For this review, take the finished solid that the model builds, in its own axes (mm). A direction names the side the tool comes from. Give positions to 0.01 mm unless a question says otherwise; leave off trailing zeros. Order: outer loops, then holes, each group sorted by start corner. A loop starts at its lowest first (then second) coordinate and runs counter-clockwise, first axis right, second up. Notation, with made-up numbers: (5, 30) - (35, 30) arc R14 ccw to (35, 35) - close; hole circle Ø6 at (54.5, -10.75). An arc over 180 degrees is marked (long way). Use a Markdown table: item, result. Add a question column.
1) We need section A-A on y = 1.55. Write out the cut boundary in (x, z).
2) Machinability: for faces 1 (the face through (8, 2, -7)), 2 (the face through (17, 2, -4)), 3 (the face through (18.5, -1, -5)), which of the approach directions +Z, -Z, +X, -X, +Y, -Y give a long, thin tool a straight path to every point of the face, cutting with its end or side? Answer none if there is none.
3) Clearance check with flat-ended pins moving along their axes: P1, Ø3, axis at x = 9, z = -13.5, coming from the -Y side; P2, Ø1, axis at y = 2, z = -6, coming from the -X side; P3, Ø5, axis at x = 13, z = -10.5, coming from the +Y side; P4, Ø0.8, axis at y = -1, z = -8, coming from the +X side. State where each tip first meets the part, or that it passes through.
4) Wall thickness on L1, parallel to Z at x = 8.5, y = 2.4; L2, parallel to X at y = 1.55, z = -5; L3, parallel to Z at x = 16.25, y = -1.8: over which ranges is each line inside the solid? List them lowest first.
5) We need section B-B on y = -0.5. Write out the cut boundary in (x, z).
6) We need section D-D on z = -13.5. Write out the cut boundary in (x, y).
7) We need section C-C on x = 19. Write out the cut boundary in (y, z).
8) Mouldability with a two-part tool opening along Z and no side actions: class faces 4 (the face through (16, -1, -8)), 5 (the face through (8, 2, -3.5)), 6 (the face through (17, -1, -7.5)) as released by +Z, released by -Z, zero draft, split by the parting line, or undercut.
```python
from build123d import *

# Parameters (mm, degrees)
SKIZZE1_W                       = 23
SKIZZE1_H                       = 19.5
AUFSATZ_LINEAR_AUSTRAGEN1_DEPTH = 1
SKIZZE2_W                       = 5
SKIZZE2_H                       = 6
AUFSATZ_LINEAR_AUSTRAGEN2_DEPTH = 2
SKIZZE3_W                       = 5
SKIZZE3_H                       = 3.5
AUFSATZ_LINEAR_AUSTRAGEN3_DEPTH = 1.5
SKIZZE4_W                       = 2.5
SKIZZE4_H                       = 1.5
AUFSATZ_LINEAR_AUSTRAGEN4_DEPTH = 2


with BuildPart() as part:
    # Skizze1 → Aufsatz-Linear austragen1 (new body)
    with BuildSketch(Plane(origin=(0, 0, 0), x_dir=(1, 0, 0), z_dir=(0, 1, 0))):
        with Locations((11.5, 9.75)):
            Rectangle(SKIZZE1_W, SKIZZE1_H)
    extrude(amount=AUFSATZ_LINEAR_AUSTRAGEN1_DEPTH)

    # Skizze2 → Aufsatz-Linear austragen2 (add)
    with BuildSketch(Plane(origin=(0, 1, 0), x_dir=(1, 0, 0), z_dir=(0, 1, 0))):
        with Locations((17.5, 7)):
            Rectangle(SKIZZE2_W, SKIZZE2_H)
    extrude(amount=AUFSATZ_LINEAR_AUSTRAGEN2_DEPTH)

    # Skizze3 → Aufsatz-Linear austragen3 (add)
    with BuildSketch(Plane(origin=(0, 1, 0), x_dir=(1, 0, 0), z_dir=(0, 1, 0))):
        with Locations((8.5, 14.25)):
            Rectangle(SKIZZE3_W, SKIZZE3_H)
        with Locations((8.5, 5.25)):
            Rectangle(SKIZZE3_W, SKIZZE3_H)
    aufsatz_linear_austragen3 = extrude(amount=AUFSATZ_LINEAR_AUSTRAGEN3_DEPTH)

    # Spiegeln1: Aufsatz-Linear austragen3 across plane
    add(aufsatz_linear_austragen3.mirror(Plane.ZX.offset(0.5)))

    # Skizze4 → Aufsatz-Linear austragen4 (add)
    with BuildSketch(Plane.XZ):
        with Locations((17.25, -8.25)):
            Rectangle(SKIZZE4_W, SKIZZE4_H)
        with Locations((17.25, -5.25)):
            Rectangle(SKIZZE4_W, SKIZZE4_H)
    extrude(amount=AUFSATZ_LINEAR_AUSTRAGEN4_DEPTH)


solid = part.part
```
Checked values:
| question | item | result |
|---|---|---|
| 1 | outline | (6, -16) - (11, -16) - (11, -12.5) - (6, -12.5) - close; (6, -7) - (11, -7) - (11, -3.5) - (6, -3.5) - close; (15, -10) - (20, -10) - (20, -4) - (15, -4) - close |
| 2 | face 1 | -X, +Y |
| 2 | face 2 | +Z, +X, +Y |
| 2 | face 3 | +Z, -Z, +X, -Y |
| 3 | P1 | y = -1.5 |
| 3 | P2 | x = 6 |
| 3 | P3 | y = 3 |
| 3 | P4 | x = 18.5 |
| 4 | L1 | -16 to -12.5, -7 to -3.5 |
| 4 | L2 | 6 to 11, 15 to 20 |
| 4 | L3 | -9 to -7.5, -6 to -4.5 |
| 5 | outline | (6, -16) - (11, -16) - (11, -12.5) - (6, -12.5) - close; (6, -7) - (11, -7) - (11, -3.5) - (6, -3.5) - close; (16, -9) - (18.5, -9) - (18.5, -7.5) - (16, -7.5) - close; (16, -6) - (18.5, -6) - (18.5, -4.5) - (16, -4.5) - close |
| 6 | outline | (0, 0) - (6, 0) - (6, -1.5) - (11, -1.5) - (11, 0) - (23, 0) - (23, 1) - (11, 1) - (11, 2.5) - (6, 2.5) - (6, 1) - (0, 1) - close |
| 7 | outline | (0, -19.5) - (1, -19.5) - (1, -10) - (3, -10) - (3, -4) - (1, -4) - (1, 0) - (0, 0) - close |
| 8 | face 4 | zero draft |
| 8 | face 5 | released by +Z |
| 8 | face 6 | undercut |
